Part model, mm, in its own coordinate system. A direction names the side the tool comes from. Give positions to 0.01 mm unless a question says otherwise; leave off trailing zeros. Loops run counter-clockwise (first coordinate to the right, second up) from the corner with the lowest first, then second, coordinate; pieces in that order, holes last. Notation, with made-up numbers: (71, 4.25) -> (114, 4.25) arc R17 ccw to (114, 19.25) -> close; hole circle Ø9 at (19, -29.5). An arc over 180 degrees is marked (long way). Write item = value, one per line.
from build123d import *

# Parameters (mm, degrees)
BOSS_EXTRUDE1_DEPTH     = 4.3
SKETCH3_W               = 10
SKETCH3_H               = 236
BOSS_EXTRUDE2_DEPTH     = 20
SKETCH4_R               = 5
BOSS_EXTRUDE3_DEPTH     = 2
FILLET1_R               = 0.5
SKETCH5_R               = 2.5
CUT_EXTRUDE1_DEPTH      = 36.5
CUT_EXTRUDE1_DEPTH_BACK = 116.5


with BuildPart() as part:
    # Sketch2 → Boss-Extrude1 (new body)
    with BuildSketch(Plane(origin=(0, 0, 0), x_dir=(1, 0, 0), z_dir=(0, 1, 0))):
        Polygon((-75.5, -118), (0, -118), (0, 118), (-65.5, 118), align=None)
        Polygon((0, 118), (0, -118), (75.5, -118), (65.5, 118), align=None)
    extrude(amount=BOSS_EXTRUDE1_DEPTH)

    # Sketch3 → Boss-Extrude2 (add)
    with BuildSketch(Plane.XZ):
        with Locations((-35, 0)):
            Rectangle(SKETCH3_W, SKETCH3_H)
        with Locations((35, 0)):
            Rectangle(SKETCH3_W, SKETCH3_H)
    extrude(amount=BOSS_EXTRUDE2_DEPTH)

    # Sketch4 → Boss-Extrude3 (add)
    with BuildSketch(Plane(origin=(0, 4.3, 0), x_dir=(1, 0, 0), z_dir=(0, 1, 0))):
        with Locations((-55.5, 108)):
            Circle(SKETCH4_R)
        with Locations((55.5, 108)):
            Circle(SKETCH4_R)
        with Locations((-55.5, -108)):
            Circle(SKETCH4_R)
        with Locations((55.5, -108)):
            Circle(SKETCH4_R)
    extrude(amount=BOSS_EXTRUDE3_DEPTH)

    # Fillet1
    fillet1_edges = [part.edges().sort_by_distance(p)[0] for p in [
        (-60.5, 6.3, -108),
        (50.5, 6.3, -108),
        (-60.5, 6.3, 108),
        (50.5, 6.3, 108),
    ]]
    fillet(fillet1_edges, radius=FILLET1_R)

    # Sketch5 → Cut-Extrude1 (cut, two sides)
    with BuildSketch(Plane.ZY.offset(40)) as cut_extrude1_sk:
        with Locations((-59, -10)):
            Circle(SKETCH5_R)
        with Locations((59, -10)):
            Circle(SKETCH5_R)
    extrude(amount=CUT_EXTRUDE1_DEPTH, mode=Mode.SUBTRACT)
    extrude(cut_extrude1_sk.sketch, amount=-CUT_EXTRUDE1_DEPTH_BACK, mode=Mode.SUBTRACT)


solid = part.part
1) Drill centre lines: line 1 along Y through (x, z) = (36, 59); line 2 along X through (y, z) = (-10.75, -41); line 3 along Y through (x, z) = (67.5, 78). Where is each one in solid material? Low to high. Write a range as [from, to].
Resolved:
line_1 = [-20, -12.5], [-7.5, 4.3]
line_2 = [-40, -30], [30, 40]
line_3 = [0, 4.3]
2) Slice it at B-B, the plane y = -10. List the corners of the cut face in (x, z), and give its area (3 significant figures).
Resolved:
outline = (-40, -118) -> (-30, -118) -> (-30, -61.5) -> (-40, -61.5) -> close; (-40, -56.5) -> (-30, -56.5) -> (-30, 56.5) -> (-40, 56.5) -> close; (-40, 61.5) -> (-30, 61.5) -> (-30, 118) -> (-40, 118) -> close; (30, -118) -> (40, -118) -> (40, -61.5) -> (30, -61.5) -> close; (30, -56.5) -> (40, -56.5) -> (40, 56.5) -> (30, 56.5) -> close; (30, 61.5) -> (40, 61.5) -> (40, 118) -> (30, 118) -> close
area = 4,520 mm²
3) Slice it at A-A, the plane z = -59. List the corners of the cut face in (x, y), and give its area (3 significant figures).
Resolved:
outline = (-68, 0) -> (-40, 0) -> (-40, -7.5) -> (-30, -7.5) -> (-30, 0) -> (30, 0) -> (30, -7.5) -> (40, -7.5) -> (40, 0) -> (68, 0) -> (68, 4.3) -> (-68, 4.3) -> close; (-40, -20) -> (-30, -20) -> (-30, -12.5) -> (-40, -12.5) -> close; (30, -20) -> (40, -20) -> (40, -12.5) -> (30, -12.5) -> close
area = 885 mm²
4) Drop flat-ended pins along their axis: P1, Ø4, axis at y = -10, z = -59, coming from the -X side; P2, Ø12, axis at y = -8, z = 22.5, coming from the +X side; P3, Ø3, axis at y = -8, z = -1, coming from the -X side; P4, Ø12, axis at x = -16.5, z = -26.5, coming from the +Y side. Give the stop position or say it passes through.
Resolved:
P1 = through
P2 = 40
P3 = -40
P4 = 4.3
5) Which spindle directions (+Z, -Z, +X, -X, +Y, -Y) get a long thin tool onto all of the face, cutting with end or side? Do faces 4 (the face through (55, 6.3, -108)), 5 (the face through (-59.185, 5.04, 104.621)), 6 (the face through (54, 0, -2)), 7 (the face through (0, 0, -2)). Say none if no direction does.
Resolved:
face_4 = +Z, -Z, +X, -X, +Y
face_5 = +Y
face_6 = +Z, -Z, +X, -Y
face_7 = +Z, -Z, -Y
6) Slice it at D-D, the plane x = -55.5. List the corners of the cut face in (y, z).
Resolved:
outline = (0, -118) -> (4.3, -118) -> (4.3, -113) -> (5.8, -113) arc R0.5 ccw to (6.3, -112.5) -> (6.3, -103.5) arc R0.5 ccw to (5.8, -103) -> (4.3, -103) -> (4.3, 103) -> (5.8, 103) arc R0.5 ccw to (6.3, 103.5) -> (6.3, 112.5) arc R0.5 ccw to (5.8, 113) -> (4.3, 113) -> (4.3, 118) -> (0, 118) -> close
7) Pull direction Z, two halves, no side cores. Call faces 1 (the face through (30, -10, -2)), 2 (the face through (-59.185, 5.04, -111.379)), 3 (the face through (0, 1, -118)): pulls with the +Z half, pulls with the -Z half, needs draft (parallel to the pull), parting line crosses it, or undercut.
Resolved:
face_1 = needs draft
face_2 = undercut
face_3 = pulls with the -Z half
8) Slice it at C-C, the plane x = 34. List the corners of the cut face in (y, z), and give its area (3 significant figures).
Resolved:
outline = (-20, -118) -> (4.3, -118) -> (4.3, 118) -> (-20, 118) -> close; hole circle Ø5 at (-10, -59); hole circle Ø5 at (-10, 59)
area = 5,700 mm²
